Build history of the part. All positions in model axes, mm. A direction names the side the tool comes from. Give positions to 0.01 mm unless a question says otherwise; leave off trailing zeros. Write each loop counter-clockwise with the first axis right and the second up, starting at its lowest first coordinate (ties: lowest second). Pieces come first, ordered by that corner, then holes. Notation, with made-up numbers: (55, 47) -> (89, 47) arc R19 cw to (89, 79) -> close; hole circle Ø7 at (78, -1). An arc over 180 degrees is marked (long way). One line per question, with ' | ' between items. Start each with the question number.
(1) Pin check, flat tips, straight feed: P1, Ø2.5, axis at x = 107, y = 10, coming from the -Z side; P2, Ø1, axis at x = 18.5, z = 57, coming from the +Y side; P3, Ø12, axis at x = 50, y = 15, coming from the -Z side. Stop position of each tip, or through.
(2) Band-saw the part on A-A, the plane z = -5.5. Give the cut face in (x, y), and give its area (3 significant figures).
(3) Band-saw the part on C-C, the plane x = -21. Give the cut face in (y, z).
(4) Band-saw the part on B-B, the plane y = 15. Give the cut face in (x, z).
(5) Tool access for faces 1 (the flat face through (105, 13, 1)), 2 (the flat face through (1, 10, 88.5)), 3 (the flat face through (-108, 13, -83.5)): list every direction of +Z, -Z, +X, -X, +Y, -Y with a clear straight run to the whole face (end or side of a thin tool).
(6) Drill centre lines: probe 1 along X at (y, z) = (10.25, 14.5); probe 2 along Y at (x, z) = (27, -40.5); probe 3 along Z at (x, y) = (-95.5, 10.5). Where is each one in solid material? Low to high. Write a range as from..to.
from build123d import *

# Parameters (mm, degrees)
SKETCH1_W           = 220
SKETCH1_H           = 177
BOSS_EXTRUDE1_DEPTH = 5
FILLET1_R           = 5
BOSS_EXTRUDE2_START = 15
BOSS_EXTRUDE2_DEPTH = 15


with BuildPart() as part:
    # Sketch1 → Boss-Extrude1 (new body)
    with BuildSketch(Plane(origin=(0, 0, 0), x_dir=(1, 0, 0), z_dir=(0, 1, 0))):
        Rectangle(SKETCH1_W, SKETCH1_H)
    extrude(amount=BOSS_EXTRUDE1_DEPTH)

    # Fillet1
    fillet1_edges = [part.edges().sort_by_distance(p)[0] for p in [
        (110, 2.5, 88.5),
        (-110, 2.5, 88.5),
    ]]
    fillet(fillet1_edges, radius=FILLET1_R)

    # Sketch3 → Boss-Extrude2 (add)
    with BuildSketch(Plane(origin=(0, 5, 0), x_dir=(1, 0, 0), z_dir=(0, 1, 0)).offset(BOSS_EXTRUDE2_START)):
        with BuildLine():
            Line((-105, 83.5), (-105, -83.5))
            Line((-105, -83.5), (105, -83.5))
            Line((105, -83.5), (105, 83.5))
            Line((105, 83.5), (110, 83.5))
            Line((110, 83.5), (110, -83.5))
            ThreePointArc((110, -83.5), (108.535533906, -87.035533906), (105, -88.5))
            Line((105, -88.5), (-105, -88.5))
            ThreePointArc((-105, -88.5), (-108.535533906, -87.035533906), (-110, -83.5))
            Line((-110, -83.5), (-110, 83.5))
            Line((-110, 83.5), (-105, 83.5))
        make_face()
    extrude(amount=-BOSS_EXTRUDE2_DEPTH)


solid = part.part
Results:
1) P1: stops at z = -83.5 | P2: stops at y = 5 | P3: stops at z = 83.5
2) outline: (-110, 0) -> (110, 0) -> (110, 20) -> (105, 20) -> (105, 5) -> (-105, 5) -> (-105, 20) -> (-110, 20) -> close | area: 1,250 mm²
3) outline: (0, -88.5) -> (5, -88.5) -> (5, 83.5) -> (20, 83.5) -> (20, 88.5) -> (0, 88.5) -> close
4) outline: (-110, -83.5) -> (-105, -83.5) -> (-105, 83.5) -> (105, 83.5) -> (105, -83.5) -> (110, -83.5) -> (110, 83.5) arc R5 ccw to (105, 88.5) -> (-105, 88.5) arc R5 ccw to (-110, 83.5) -> close
5) face 1: -Z, +Y | face 2: +Z, +X, -X, +Y, -Y | face 3: -Z, +X, -X, +Y
6) probe 1: x = -110..-105, 105..110 | probe 2: y = 0..5 | probe 3: z = 83.5..88.5
